Check sheet for the modelled part. Datum: model origin and axes. Units: mm. Face numbers are marked on the shaded views. A direction names the side the tool comes from. Give positions to 0.01 mm unless a question says otherwise; leave off trailing zeros. Write each loop counter-clockwise with the first axis right and the second up, starting at its lowest first coordinate (ties: lowest second). Pieces come first, ordered by that corner, then holes. Notation, with made-up numbers: M 68,76 L 74,76 A20 ccw 74,86 Z; hole C 66.25,-1.75 d3. An arc over 180 degrees is marked long. Write item = value, one per line. Start each with the question number.
1) Sectioned sample at B-B, the plane x = -1.5. Record the cut outline in (y, z), then the cut area to 3 significant figures.
2) Sectioned sample at D-D, the plane z = 4. Record the cut outline in (x, y).
3) Sectioned sample at A-A, the plane z = -65.5. Record the cut outline in (x, y), then the cut area to 3 significant figures.
4) Sectioned sample at C-C, the plane y = -16.75. Record the cut outline in (x, z).
5) Gauge pin test, flat ends, axial feed: pin 1 (4 mm diameter, centred on x = -6.5, y = -13, fed in from -Z); pin 2 (2 mm diameter, centred on x = -7.5, z = -30, fed in from +Y); pin 3 (6 mm diameter, centred on x = 4, z = -41, fed in from +Y). Record the tip position at first contact, or that the pin passes through.
6) Scan lines: L1, parallel to Z at x = -2.5, y = -0.25; L2, parallel to Z at x = 8, y = -3.5; L3, parallel to Y at x = 4.75, z = -73. Record each from-to range of solid material in increasing order.
7) Set-up check for the marked faces 1 and 2: record each of +Z, -Z, +X, -X, +Y, -Y from which the full face is reachable in a straight line by a thin tool's end or side.
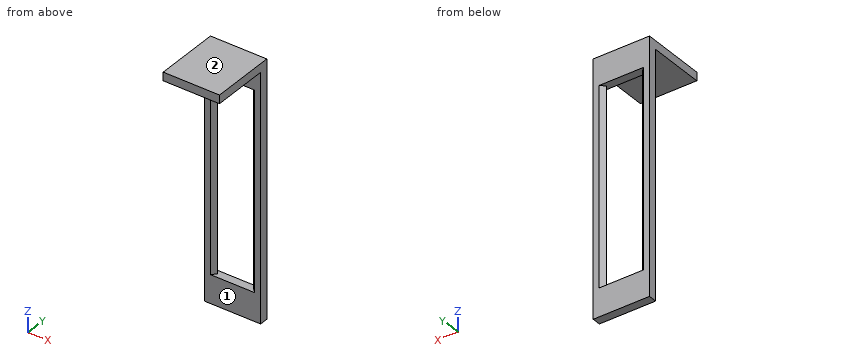
from build123d import *

# Parameters (mm, degrees)
SKETCH_W     = 20
SKETCH_H     = 3
PAD_DEPTH    = 10
PAD001_DEPTH = 70
SKETCH002_W  = 20
SKETCH002_H  = 3
PAD002_DEPTH = 10
SKETCH006_W  = 20
SKETCH006_H  = 3
PAD004_DEPTH = 20


with BuildPart() as part:
    # Sketch (on XY_Plane of Origin) → Pad (new body)
    with BuildSketch(Plane.XY):
        Rectangle(SKETCH_W, SKETCH_H)
    extrude(amount=PAD_DEPTH)

    # Sketch001 (on Face5 of Pad) → Pad001 (join)
    with BuildSketch(Plane(origin=(0, 0, 0), x_dir=(1, 0, 0), z_dir=(0, 0, -1))):
        Polygon((-7.87868, 1.5), (-6.37868, 0), (-7.87868, -1.5), (-10, -1.5), (-10, 1.5), align=None)
        Polygon((7.87868, 1.5), (6.37868, 0), (7.87868, -1.5), (10, -1.5), (10, 1.5), align=None)
    extrude(amount=PAD001_DEPTH)

    # Sketch002 (on Face7 of Pad001) → Pad002 (join)
    with BuildSketch(Plane(origin=(0, 0, -70), x_dir=(1, 0, 0), z_dir=(0, 0, -1))):
        Rectangle(SKETCH002_W, SKETCH002_H)
    extrude(amount=PAD002_DEPTH)

    # Sketch006 (on Face10 of Pad002) → Pad004 (join)
    with BuildSketch(Plane.XZ.offset(1.5)):
        with Locations((0, 8.5)):
            Rectangle(SKETCH006_W, SKETCH006_H)
    extrude(amount=PAD004_DEPTH)


solid = part.part
Data:
q1.outline = M -21.5,7 L -1.5,7 L -1.5,0 L 1.5,0 L 1.5,10 L -21.5,10 Z; M -1.5,-80 L 1.5,-80 L 1.5,-70 L -1.5,-70 Z
q1.area = 120 mm2
q2.outline = M -10,-1.5 L 10,-1.5 L 10,1.5 L -10,1.5 Z
q3.outline = M -10,-1.5 L -7.88,-1.5 L -6.38,0 L -7.88,1.5 L -10,1.5 Z; M 6.38,0 L 7.88,-1.5 L 10,-1.5 L 10,1.5 L 7.88,1.5 Z
q3.area = 17.2 mm2
q4.outline = M -10,7 L 10,7 L 10,10 L -10,10 Z
q5.pin_1 = 7
q5.pin_2 = 1.5
q5.pin_3 = 0.62
q6.L1 = -80 to -70, 0 to 10
q6.L2 = 7 to 10
q6.L3 = -1.5 to 1.5
q7.face_1 = -Z, +X, -X, -Y
q7.face_2 = +Z, +X, -X, +Y, -Y
